Part model, mm, in its own coordinate system. Face numbers are marked on the shaded views. Coordinates: 2 decimals unless noted, no trailing zeros. Write each loop counter-clockwise with the first axis right and the second up, starting at its lowest first coordinate (ties: lowest second). Pieces come first, ordered by that corner, then holes. Notation, with made-up numbers: (42.5, 4.25) -> (75.5, 4.25) arc R17 ccw to (75.5, 24.25) -> close; hole circle Ø11 at (-39, 37). An arc over 180 degrees is marked (long way). Write item = value, one per line.
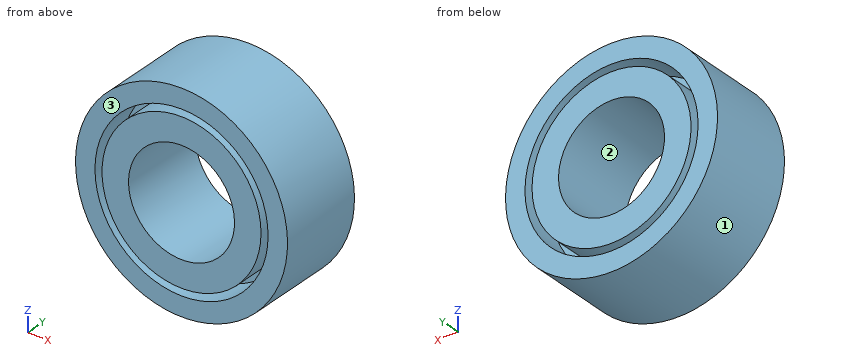
from build123d import *

# Parameters (mm, degrees)
SKETCH_1_R          = 3
SKETCH_1_R_2        = 1.5
EXTRUDE_1_DEPTH     = 2.5
SKETCH_1_3_R        = 2.45
SKETCH_1_3_R_2      = 2.25
CUT_EXTRUDE_1_DEPTH = 1
CUT_EXTRUDE_START   = 1.5
SKETCH_1_4_R        = 2.45
SKETCH_1_4_R_2      = 2.25
CUT_EXTRUDE_2_DEPTH = 1


with BuildPart() as part:
    # 草图1 → 凸台-拉伸1 (new body)
    with BuildSketch(Plane(origin=(0, 0, 0), x_dir=(1, 0, 0), z_dir=(0, 1, 0))):
        with Locations(Location((0, 0, 0), (0, 0, 270))):
            Circle(SKETCH_1_R)
        with Locations(Location((0, 0, 0), (0, 0, 270))):
            Circle(SKETCH_1_R_2, mode=Mode.SUBTRACT)
    extrude(amount=EXTRUDE_1_DEPTH)

    # 草图1<3> → 切除-拉伸-薄壁1 (cut)
    with BuildSketch(Plane(origin=(0, 0, 0), x_dir=(1, 0, 0), z_dir=(0, 1, 0))):
        Circle(SKETCH_1_3_R)
        Circle(SKETCH_1_3_R_2, mode=Mode.SUBTRACT)
    extrude(amount=CUT_EXTRUDE_1_DEPTH, mode=Mode.SUBTRACT)

    # 草图1<4> → 切除-拉伸-薄壁2 (cut)
    with BuildSketch(Plane(origin=(0, 0, 0), x_dir=(1, 0, 0), z_dir=(0, 1, 0)).offset(CUT_EXTRUDE_START)):
        Circle(SKETCH_1_4_R)
        Circle(SKETCH_1_4_R_2, mode=Mode.SUBTRACT)
    extrude(amount=CUT_EXTRUDE_2_DEPTH, mode=Mode.SUBTRACT)


solid = part.part
Q1. Mould opens along X. For the marked faces 1, 2 and 3 say: released by +X, released by -X, zero draft, split by the parting line, or undercut.
Model answer:
face_1 = split by the parting line
face_2 = undercut
face_3 = zero draft
Q2. Saw through at C-C on y = 0.75. Give the cut face in (x, z), and give its area (3 significant figures).
Model answer:
outline = circle Ø6 at (0, 0); circle Ø4.5 at (0, 0); hole circle Ø4.9 at (0, 0); hole circle Ø3 at (0, 0)
area = 18.3 mm²
Q3. Saw through at A-A on z = 0. Give the cut face in (x, y).
Model answer:
outline = (-3, 0) -> (-2.45, 0) -> (-2.45, 1) -> (-2.25, 1) -> (-2.25, 0) -> (-1.5, 0) -> (-1.5, 2.5) -> (-2.25, 2.5) -> (-2.25, 1.5) -> (-2.45, 1.5) -> (-2.45, 2.5) -> (-3, 2.5) -> close; (1.5, 0) -> (2.25, 0) -> (2.25, 1) -> (2.45, 1) -> (2.45, 0) -> (3, 0) -> (3, 2.5) -> (2.45, 2.5) -> (2.45, 1.5) -> (2.25, 1.5) -> (2.25, 2.5) -> (1.5, 2.5) -> close
Q4. Pin check, flat tips, straight feed: pin 1 (1.5 mm diameter, centred on x = 1, z = 0.5, fed in from +Y); pin 2 (1 mm diameter, centred on y = 0.5, z = -1, fed in from -X). Stop position of each tip, or through.
Model answer:
pin_1 = 2.5
pin_2 = -2.96
Q5. Probe line 1 (X direction, y = 2, z = 0); line 2 (X direction, y = 0.6, z = 1.1); line 3 (Z direction, x = -0.5, y = 0.7). List the from-to ranges inside material, lowest first. Write a range as from..to.
Model answer:
line_1 = -3..-2.45, -2.25..-1.5, 1.5..2.25, 2.45..3
line_2 = -2.79..-2.19, -1.96..-1.02, 1.02..1.96, 2.19..2.79
line_3 = -2.96..-2.4, -2.19..-1.41, 1.41..2.19, 2.4..2.96
Q6. Saw through at B-B on x = 0. Give the cut face in (y, z).
Model answer:
outline = (0, -3) -> (2.5, -3) -> (2.5, -2.45) -> (1.5, -2.45) -> (1.5, -2.25) -> (2.5, -2.25) -> (2.5, -1.5) -> (0, -1.5) -> (0, -2.25) -> (1, -2.25) -> (1, -2.45) -> (0, -2.45) -> close; (0, 1.5) -> (2.5, 1.5) -> (2.5, 2.25) -> (1.5, 2.25) -> (1.5, 2.45) -> (2.5, 2.45) -> (2.5, 3) -> (0, 3) -> (0, 2.45) -> (1, 2.45) -> (1, 2.25) -> (0, 2.25) -> close
Q7. Saw through at D-D on y = 1.1. Give the cut face in (x, z), and give its area (3 significant figures).
Model answer:
outline = circle Ø6 at (0, 0); hole circle Ø3 at (0, 0)
area = 21.2 mm²
